The listing builds one solid part. Answer for the finished solid, in the listing's coordinates (mm). A direction names the side the tool comes from. Coordinates: 2 decimals unless noted, no trailing zeros. Order: outer loops, then holes, each group sorted by start corner. A loop starts at its lowest first (then second) coordinate and runs counter-clockwise, first axis right, second up. Notation, with made-up numbers: (33, 12) -> (75, 12) arc R20 ccw to (75, 30) -> close; hole circle Ø4 at (-3, 4). An arc over 180 degrees is marked (long way). Answer in a Markdown table with one row per item.
```python
from build123d import *

# Parameters (mm, degrees)
SKETCH1_W                      = 14.7
SKETCH1_H                      = 14.7
BOSS_EXTRUDE1_DEPTH            = 87.63
BOSS_EXTRUDE1_2_DEPTH          = 87.63
SKETCH2_W                      = 95.44
SKETCH2_H                      = 44.45
BOSS_EXTRUDE2_DEPTH            = 2.54
CHAMFER2_SIZE                  = 2
SKETCH12_W                     = 50.8
SKETCH12_H                     = 44.45
BOSS_EXTRUDE5_DEPTH            = 13.97
SKETCH3_R                      = 17.78
SKETCH3_R_2                    = 1.6
CUT_EXTRUDE1_DEPTH             = 107.454804025
BOSS_EXTRUDE3_DEPTH            = 5.08
BOSS_EXTRUDE3_DEPTH_BACK       = 10.16
SKETCH4_W                      = 50.8
SKETCH4_H                      = 3.81
SKETCH5_W                      = 5.08
SKETCH5_H                      = 24.13
BOSS_EXTRUDE4_DEPTH            = 31.75
SKETCH6_R                      = 3.175
TRAYSUPPORTMOUNTINGHOLES_DEPTH = 135.547891102
SKETCH11_R                     = 3.175
CUT_EXTRUDE5_DEPTH             = 124.012238822
CHAMFER4_SIZE                  = 1
CUT_EXTRUDE6_START             = -11.43
SKETCH13_W                     = 43.18
SKETCH13_H                     = 40.64
CUT_EXTRUDE6_DEPTH             = 11.43
SKETCH15_W                     = 22.32
SKETCH15_H                     = 44.45
BOSS_EXTRUDE6_DEPTH            = 13.97
CUT_EXTRUDE7_DEPTH             = 135.547891102
CUT_EXTRUDE8_DEPTH             = 122.229277817
CUT_EXTRUDE9_DEPTH             = 115.023552392
CHAMFER5_SIZE                  = 2.54
CHAMFER6_SIZE                  = 2.54
SKETCH22_W                     = 48.26
SKETCH22_H                     = 41.79
SKETCH22_R                     = 1.905
SKETCH22_R_2                   = 19.75
BOSS_EXTRUDE7_DEPTH            = 14.8


with BuildPart() as part:
    # Sketch1 → Boss-Extrude1 (new body)
    with BuildSketch(Plane(origin=(0, 0, 0), x_dir=(1, 0, 0), z_dir=(0, 1, 0))):
        with Locations((40.37, 0)):
            Rectangle(SKETCH1_W, SKETCH1_H)
    extrude(amount=BOSS_EXTRUDE1_DEPTH)



with BuildPart() as body_2:
    # Sketch1 → Boss-Extrude1 2 (new body)
    with BuildSketch(Plane(origin=(0, 0, 0), x_dir=(1, 0, 0), z_dir=(0, 1, 0))):
        with Locations((-40.37, 0)):
            Rectangle(SKETCH1_W, SKETCH1_H)
    extrude(amount=BOSS_EXTRUDE1_2_DEPTH)


with BuildPart() as part_1:
    add(part.part)

    add(body_2.part)  # Boss-Extrude2 merges body 2
    # Sketch2 → Boss-Extrude2 (add)
    with BuildSketch(Plane(origin=(0, 87.63, 0), x_dir=(1, 0, 0), z_dir=(0, 1, 0))):
        with Locations((0, -14.875)):
            Rectangle(SKETCH2_W, SKETCH2_H)
    extrude(amount=-BOSS_EXTRUDE2_DEPTH)

    # Chamfer2
    chamfer2_edges = [part_1.edges().sort_by_distance(p)[0] for p in [
        (-47.72, 0, 0),
        (-33.02, 0, 0),
        (-40.37, 0, 7.35),
        (-40.37, 0, -7.35),
        (40.37, 0, -7.35),
        (47.72, 0, 0),
        (40.37, 0, 7.35),
        (33.02, 0, 0),
    ]]
    chamfer(chamfer2_edges, length=CHAMFER2_SIZE)

    # Sketch12 → Boss-Extrude5 (add)
    with BuildSketch(Plane.XZ.offset(-85.09)):
        with Locations((0, 14.875)):
            Rectangle(SKETCH12_W, SKETCH12_H)
    extrude(amount=BOSS_EXTRUDE5_DEPTH)

    # Sketch3 → Cut-Extrude1 (cut, through all)
    with BuildSketch(Plane(origin=(0, 87.63, 0), x_dir=(1, 0, 0), z_dir=(0, 1, 0))):
        with Locations(Location((0, -12.15, 0), (0, 0, 270))):
            Circle(SKETCH3_R)
        with Locations(Location((-15.5, 3.35, 0), (0, 0, 270))):
            Circle(SKETCH3_R_2)
        with Locations(Location((-15.5, -27.65, 0), (0, 0, 270))):
            Circle(SKETCH3_R_2)
        with Locations(Location((15.5, -27.65, 0), (0, 0, 270))):
            Circle(SKETCH3_R_2)
        with Locations(Location((15.5, 3.35, 0), (0, 0, 270))):
            Circle(SKETCH3_R_2)
    extrude(amount=-CUT_EXTRUDE1_DEPTH, mode=Mode.SUBTRACT)

    # Sketch4 → Boss-Extrude3 (add, two sides: drawn at the far end of the back side and taken through both)
    with BuildSketch(Plane.XZ.offset(-85.09).offset(-BOSS_EXTRUDE3_DEPTH_BACK)):
        with Locations((0, 35.195)):
            Rectangle(SKETCH4_W, SKETCH4_H)
    extrude(amount=BOSS_EXTRUDE3_DEPTH + BOSS_EXTRUDE3_DEPTH_BACK)

    # Sketch5 → Boss-Extrude4 (add)
    with BuildSketch(Plane.XY.offset(37.1)):
        with Locations((-15.24, 83.185)):
            Rectangle(SKETCH5_W, SKETCH5_H)
        with Locations((15.24, 83.185)):
            Rectangle(SKETCH5_W, SKETCH5_H)
    extrude(amount=BOSS_EXTRUDE4_DEPTH)

    # Sketch6 → TraySupportMountingHoles (cut, through all)
    with BuildSketch(Plane.ZY.offset(17.78)):
        with Locations(Location((49.165, 88.9, 0), (0, 0, 270))):
            Circle(SKETCH6_R)
        with Locations(Location((60.595, 88.9, 0), (0, 0, 270))):
            Circle(SKETCH6_R)
    extrude(amount=-TRAYSUPPORTMOUNTINGHOLES_DEPTH, mode=Mode.SUBTRACT)

    # Sketch11 → Cut-Extrude5 (cut, through all)
    with BuildSketch(Plane.XY.offset(7.35)):
        with Locations((-40.37, 65.405)):
            Circle(SKETCH11_R)
        with Locations((-40.37, 51.435)):
            Circle(SKETCH11_R)
        with Locations((-40.37, 37.465)):
            Circle(SKETCH11_R)
        with Locations((-40.37, 23.495)):
            Circle(SKETCH11_R)
        with Locations((-40.37, 9.525)):
            Circle(SKETCH11_R)
    cut_extrude5 = extrude(amount=-CUT_EXTRUDE5_DEPTH, mode=Mode.SUBTRACT)

    # Mirror1: Cut-Extrude5 across plane
    add(cut_extrude5.mirror(Plane(origin=(0, 0, 0), x_dir=(0, 0, 1), z_dir=(1, 0, 0))), mode=Mode.SUBTRACT)

    # Chamfer4
    chamfer4_edges = [part_1.edges().sort_by_distance(p)[0] for p in [
        (-43.545, 65.405, -7.35),
        (-43.545, 65.405, 7.35),
        (-43.545, 23.495, -7.35),
        (-43.545, 23.495, 7.35),
        (-43.545, 37.465, -7.35),
        (-43.545, 37.465, 7.35),
        (-43.545, 51.435, -7.35),
        (-43.545, 51.435, 7.35),
        (-43.545, 9.525, -7.35),
        (-43.545, 9.525, 7.35),
        (43.545, 65.405, 7.35),
        (43.545, 65.405, -7.35),
        (43.545, 23.495, 7.35),
        (43.545, 23.495, -7.35),
        (43.545, 37.465, 7.35),
        (43.545, 37.465, -7.35),
        (43.545, 51.435, 7.35),
        (43.545, 51.435, -7.35),
        (43.545, 9.525, 7.35),
        (43.545, 9.525, -7.35),
    ]]
    chamfer(chamfer4_edges, length=CHAMFER4_SIZE)

    # Sketch13 → Cut-Extrude6 (cut)
    with BuildSketch(Plane(origin=(0, 87.63, 0), x_dir=(1, 0, 0), z_dir=(0, 1, 0)).offset(CUT_EXTRUDE6_START)):
        with Locations((0, -12.97)):
            Rectangle(SKETCH13_W, SKETCH13_H)
    extrude(amount=CUT_EXTRUDE6_DEPTH, mode=Mode.SUBTRACT)

    # Sketch15 → Boss-Extrude6 (add)
    with BuildSketch(Plane.XZ.offset(-85.09)):
        with Locations((36.56, 14.875)):
            Rectangle(SKETCH15_W, SKETCH15_H)
        with Locations((-36.56, 14.875)):
            Rectangle(SKETCH15_W, SKETCH15_H)
    extrude(amount=BOSS_EXTRUDE6_DEPTH)

    # Sketch17 → Cut-Extrude7 (cut, through all)
    with BuildSketch(Plane.ZY.offset(17.78)):
        Polygon((37.1, 71.12), (68.85, 84.148095119), (68.85, 71.12), align=None)
    extrude(amount=-CUT_EXTRUDE7_DEPTH, mode=Mode.SUBTRACT)

    # Sketch20 → Cut-Extrude8 (cut, through all)
    with BuildSketch(Plane(origin=(0, 87.63, 0), x_dir=(-1, 0, 0), z_dir=(0, -1, 0))):
        Polygon((-25.4, -37.1), (-47.72, -7.35), (-47.72, -37.1), align=None)
        Polygon((47.72, -7.35), (25.4, -37.1), (47.72, -37.1), align=None)
    extrude(amount=CUT_EXTRUDE8_DEPTH, mode=Mode.SUBTRACT)

    # Sketch21 → Cut-Extrude9 (cut, through all)
    with BuildSketch(Plane(origin=(0, 0, 33.29), x_dir=(-1, 0, 0), z_dir=(0, 0, -1))):
        Polygon((-25.4, 87.63), (-17.78, 95.25), (-25.4, 95.25), align=None)
        Polygon((25.4, 87.63), (17.78, 95.25), (25.4, 95.25), align=None)
    extrude(amount=-CUT_EXTRUDE9_DEPTH, mode=Mode.SUBTRACT)

    # Chamfer5
    chamfer5_edges = [part_1.edges().sort_by_distance(p)[0] for p in [
        (0, 71.12, 37.1),
        (-21.59, 71.12, 37.1),
        (34.655, 87.63, -7.35),
        (-47.72, 87.63, 0),
        (-34.655, 87.63, -7.35),
        (-21.59, 87.63, 12.97),
        (21.59, 87.63, 12.97),
        (-21.59, 81.915, -7.35),
        (21.59, 81.915, -7.35),
        (21.59, 71.12, 37.1),
        (47.72, 87.63, 0),
    ]]
    chamfer(chamfer5_edges, length=CHAMFER5_SIZE)

    # Chamfer6
    chamfer6_edges = [part_1.edges().sort_by_distance(p)[0] for p in [
        (37.512820168, 71.12, 20.955),
        (-37.512820168, 71.12, 20.955),
    ]]
    chamfer(chamfer6_edges, length=CHAMFER6_SIZE)

    # Sketch22 → Boss-Extrude7 (add)
    with BuildSketch(Plane(origin=(0, 85.92, 0), x_dir=(1, 0, 0), z_dir=(0, 1, 0))):
        with Locations((0, -12.395)):
            Rectangle(SKETCH22_W, SKETCH22_H)
        with Locations(Location((-15.5, 3.35, 0), (0, 0, 270))):
            Circle(SKETCH22_R, mode=Mode.SUBTRACT)
        with Locations(Location((15.5, 3.35, 0), (0, 0, 270))):
            Circle(SKETCH22_R, mode=Mode.SUBTRACT)
        with Locations(Location((15.5, -27.65, 0), (0, 0, 270))):
            Circle(SKETCH22_R, mode=Mode.SUBTRACT)
        with Locations(Location((-15.5, -27.65, 0), (0, 0, 270))):
            Circle(SKETCH22_R, mode=Mode.SUBTRACT)
        with Locations(Location((0, -12.15, 0), (0, 0, 270))):
            Circle(SKETCH22_R_2, mode=Mode.SUBTRACT)
    extrude(amount=-BOSS_EXTRUDE7_DEPTH)


solid = part_1.part
```
(1) A cutting plane is placed at D-D, the plane x = -15.5. Count the separate pieces of the cut face and the enclosed holes in it, then the cut area to 3 significant figures.
Check values:
| item | result |
|---|---|
| separate pieces | 4 |
| enclosed holes | 2 |
| area | 773 mm² |
(2) For a pull along X with two mould halves and no side action, classify faces 1 (the flat face through (35.715, 72.408, 21.265)), 2 (the flat face through (-21.64, 91.39, 35.17)), 3 (the cylindrical face through (-17.36, 81.13, -3.76)) as released by +X, released by -X, zero draft, split by the parting line, or undercut.
Check values:
| item | result |
|---|---|
| face 1 | released by +X |
| face 2 | released by -X |
| face 3 | undercut |
(3) A cutting plane is placed at B-B, the plane y = 58. Determine the outline of the cut face in (x, z).
Check values:
| item | result |
|---|---|
| outline | (-47.72, -7.35) -> (-33.02, -7.35) -> (-33.02, 7.35) -> (-47.72, 7.35) -> close; (33.02, -7.35) -> (47.72, -7.35) -> (47.72, 7.35) -> (33.02, 7.35) -> close |
(4) A cutting plane is placed at C-C, the plane y = 88.9. Determine the outline of the cut face in (x, z), then the cut area to 3 significant figures.
Check values:
| item | result |
|---|---|
| outline | (-24.13, 33.29) -> (24.13, 33.29) -> (24.13, 37.1) -> (17.78, 37.1) -> (17.78, 45.99) -> (12.7, 45.99) -> (12.7, 37.1) -> (-12.7, 37.1) -> (-12.7, 45.99) -> (-17.78, 45.99) -> (-17.78, 37.1) -> (-24.13, 37.1) -> close; (-17.78, 52.34) -> (-12.7, 52.34) -> (-12.7, 57.42) -> (-17.78, 57.42) -> close; (-17.78, 63.77) -> (-12.7, 63.77) -> (-12.7, 68.85) -> (-17.78, 68.85) -> close; (12.7, 52.34) -> (17.78, 52.34) -> (17.78, 57.42) -> (12.7, 57.42) -> close; (12.7, 63.77) -> (17.78, 63.77) -> (17.78, 68.85) -> (12.7, 68.85) -> close |
| area | 377 mm² |
(5) A cutting plane is placed at A-A, the plane x = 0. Determine the outline of the cut face in (y, z), then the cut area to 3 significant figures.
Check values:
| item | result |
|---|---|
| outline | (71.12, -8.5) -> (85.92, -8.5) -> (85.92, -7.6) -> (71.12, -7.6) -> close; (71.12, -7.35) -> (76.2, -7.35) -> (76.2, -5.63) -> (71.12, -5.63) -> close; (71.12, 29.93) -> (76.2, 29.93) -> (76.2, 31.9) -> (85.92, 31.9) -> (85.92, 33.29) -> (95.25, 33.29) -> (95.25, 37.1) -> (73.66, 37.1) -> (71.12, 34.56) -> close |
| area | 141 mm² |
(6) Which of the six approach directions +Z, -Z, +X, -X, +Y, -Y give full straight-line access (tool end or side, diameter ignored) to faces 4 (the flat face through (22, 82, 37.1)), 5 (the cylindrical face through (-16.66, 81.13, 26.14)), 6 (the flat face through (-15, 90, 68.85))?
Check values:
| item | result |
|---|---|
| face 4 | +Z, +X, +Y, -Y |
| face 5 | +Y |
| face 6 | +Z, +X, -X, +Y, -Y |
(7) Flat-ended cylindrical pins translate along their axes: pin 1 (4 mm diameter, centred on x = -21.5, y = 89, fed in from +Z); pin 2 (4 mm diameter, centred on x = 15.5, z = 27, fed in from +Y); pin 3 (7 mm diameter, centred on x = -41.5, y = 50.5, fed in from -Z). Find the tip coordinate at first contact, or state that the pin passes through.
Check values:
| item | result |
|---|---|
| pin 1 | z = 37.1 |
| pin 2 | y = 85.92 |
| pin 3 | z = -7.35 |
(8) Find the intervals of material crossed by line 1 along Y through (x, z) = (40.37, -1); line 2 along Y through (x, z) = (40, -3); line 3 along Z through (x, y) = (16, 88.9), in increasing order. Write a range as from..to.
Check values:
| item | result |
|---|---|
| line 1 | 0..6.35, 12.7..20.32, 26.67..34.29, 40.64..48.26, 54.61..62.23, 68.58..87.63 |
| line 2 | 0..6.37, 12.68..20.34, 26.65..34.31, 40.62..48.28, 54.59..62.25, 68.56..87.63 |
| line 3 | 33.29..45.99, 52.34..57.42, 63.77..68.85 |
